```python
from build123d import *

# Parameters (mm, degrees)
SKETCH1_R           = 47
BOSS_EXTRUDE1_DEPTH = 16
SKETCH2_R           = 44.8
CUT_EXTRUDE1_DEPTH  = 13.8
FILLET1_R           = 1.1
FILLET2_R           = 1.1


with BuildPart() as part:
    # Sketch1 → Boss-Extrude1 (new body)
    with BuildSketch(Plane(origin=(0, 0, 0), x_dir=(1, 0, 0), z_dir=(0, 1, 0))):
        with Locations(Location((0, 0, 0), (0, 0, 270))):
            Circle(SKETCH1_R)
    extrude(amount=BOSS_EXTRUDE1_DEPTH)

    # Sketch2 → Cut-Extrude1 (cut)
    with BuildSketch(Plane(origin=(0, 16, 0), x_dir=(1, 0, 0), z_dir=(0, 1, 0))):
        with Locations(Location((0, 0, 0), (0, 0, 270))):
            Circle(SKETCH2_R)
    extrude(amount=-CUT_EXTRUDE1_DEPTH, mode=Mode.SUBTRACT)

    # Fillet1
    fillet1_edges = [part.edges().sort_by_distance(p)[0] for p in [
        (0, 16, -47),
        (0, 16, -44.8),
    ]]
    fillet(fillet1_edges, radius=FILLET1_R - 0.0001)  # a hair under: the kernel refuses the full size

    # Fillet2
    fillet2_edges = [part.edges().sort_by_distance(p)[0] for p in [
        (0, 0, -47),
    ]]
    fillet(fillet2_edges, radius=FILLET2_R)


solid = part.part
```
Model file for the job. Use its own axes, mm. Round coordinates to 2 decimals unless told otherwise and drop trailing zeros. Order: outer loops, then holes, each group sorted by start corner. A loop starts at its lowest first (then second) coordinate and runs counter-clockwise, first axis right, second up. Notation, with made-up numbers: M 89.25,-7 L 106.25,-7 A33 ccw 106.25,23 Z; hole C 49,62 d4. An arc over 180 degrees is marked long. Use CSV: the item, a comma, the result in double quotes.
Item 1: Pull direction Z, two halves, no side cores. Call faces 1 (the face through (31.765, 7.903, -34.641)), 2 (the face through (1, 2.2, -1)), 3 (the face through (1, 0, -1)): released by +Z, released by -Z, zero draft, split by the parting line, or undercut.
Worked answers:
face 1,"split by the parting line"
face 2,"undercut"
face 3,"zero draft"
Item 2: Saw through at C-C (y = 11.25). List the corners of the cut face in (x, z), plus the area to 3 significant figures.
Worked answers:
outline,"C 0,0 d94; hole C 0,0 d89.6"
area,"634 mm²"
Item 3: Probe probe 1 along X at (y, z) = (9.75, -1); probe 2 along Y at (x, z) = (18.5, -28); probe 3 along X at (y, z) = (13.5, -15.5). List the from-to ranges inside material, lowest first.
Worked answers:
probe 1,"-46.99 to -44.79, 44.79 to 46.99"
probe 2,"0 to 2.2"
probe 3,"-44.37 to -42.03, 42.03 to 44.37"
Item 4: Pin check, flat tips, straight feed: pin 1 (3 mm diameter, centred on x = -7.5, z = -27.5, fed in from +Y); pin 2 (8 mm diameter, centred on x = -6.5, y = 10.5, fed in from -Z); pin 3 (6 mm diameter, centred on x = -13, y = 13, fed in from +Z). Stop position of each tip, or through.
Worked answers:
pin 1,"y = 2.2"
pin 2,"z = -46.93"
pin 3,"z = 45.92"
